Geometry check sheet. Reference: the model listing, model coordinates, mm. Face numbers are marked on the shaded views. A direction names the side the tool comes from. Round coordinates to 2 decimals unless told otherwise and drop trailing zeros. Loops run counter-clockwise (first coordinate to the right, second up) from the corner with the lowest first, then second, coordinate; pieces in that order, holes last. Notation, with made-up numbers: M -17,36 L 2,36 A21 cw 2,53 Z; hole C 40.25,1.5 d3. An arc over 180 degrees is marked long. Write item = value, one per line.
from build123d import *

# Parameters (mm, degrees)
BOSS_EXTRUDE5_DEPTH    = 10
BOSS_EXTRUDE5_2_DEPTH  = 10
BOSS_EXTRUDE5_3_DEPTH  = 10
BOSS_EXTRUDE5_4_DEPTH  = 10
BOSS_EXTRUDE5_5_DEPTH  = 10
BOSS_EXTRUDE5_6_DEPTH  = 10
BOSS_EXTRUDE5_7_DEPTH  = 10
BOSS_EXTRUDE5_8_DEPTH  = 10
BOSS_EXTRUDE5_9_DEPTH  = 10
BOSS_EXTRUDE5_10_DEPTH = 10
BOSS_EXTRUDE5_11_DEPTH = 10
BOSS_EXTRUDE5_12_DEPTH = 10
SKETCH5_W              = 13.85640646
SKETCH5_H              = 26
SKETCH5_W_2            = 26.92820323
SKETCH5_H_2            = 12
BOSS_EXTRUDE8_DEPTH    = 76.2
BOSS_EXTRUDE9_REACH    = 266.711
SKETCH9_W              = 6.35
SKETCH9_H              = 128.000000074
SKETCH9_W_2            = 11.02820323
BOSS_EXTRUDE10_DEPTH   = 152.4
SKETCH11_W             = 226.92820323
SKETCH11_H             = 76.2
BOSS_EXTRUDE11_DEPTH   = 6.35


with BuildPart() as part:
    # Sketch2 → Boss-Extrude5 (new body)
    with BuildSketch(Plane.XY):
        Polygon((-111.732050808, 13), (-113.464101615, 10), (-111.732050808, 7), (-108.267949192, 7), (-106.535898385, 10), (-108.267949192, 13), align=None)
    extrude(amount=-BOSS_EXTRUDE5_DEPTH)



with BuildPart() as body_2:
    # Sketch2 → Boss-Extrude5 2 (new body)
    with BuildSketch(Plane.XY):
        Polygon((-111.732050808, 23), (-113.464101615, 20), (-111.732050808, 17), (-108.267949192, 17), (-106.535898385, 20), (-108.267949192, 23), align=None)
    extrude(amount=-BOSS_EXTRUDE5_2_DEPTH)


with BuildPart() as body_3:
    # Sketch2 → Boss-Extrude5 3 (new body)
    with BuildSketch(Plane.XY):
        Polygon((-111.732050808, 33), (-113.464101615, 30), (-111.732050808, 27), (-108.267949192, 27), (-106.535898385, 30), (-108.267949192, 33), align=None)
    extrude(amount=-BOSS_EXTRUDE5_3_DEPTH)


with BuildPart() as body_4:
    # Sketch2 → Boss-Extrude5 4 (new body)
    with BuildSketch(Plane.XY):
        Polygon((111.732050808, 27), (113.464101615, 30), (111.732050808, 33), (108.267949192, 33), (106.535898385, 30), (108.267949192, 27), align=None)
    extrude(amount=-BOSS_EXTRUDE5_4_DEPTH)


with BuildPart() as body_5:
    # Sketch2 → Boss-Extrude5 5 (new body)
    with BuildSketch(Plane.XY):
        Polygon((111.732050808, 17), (113.464101615, 20), (111.732050808, 23), (108.267949192, 23), (106.535898385, 20), (108.267949192, 17), align=None)
    extrude(amount=-BOSS_EXTRUDE5_5_DEPTH)


with BuildPart() as body_6:
    # Sketch2 → Boss-Extrude5 6 (new body)
    with BuildSketch(Plane.XY):
        Polygon((111.732050808, 7), (113.464101615, 10), (111.732050808, 13), (108.267949192, 13), (106.535898385, 10), (108.267949192, 7), align=None)
    extrude(amount=-BOSS_EXTRUDE5_6_DEPTH)


with BuildPart() as body_7:
    # Sketch2 → Boss-Extrude5 7 (new body)
    with BuildSketch(Plane.XY):
        Polygon((61.732050808, 107), (63.464101615, 110), (61.732050808, 113), (58.267949192, 113), (56.535898385, 110), (58.267949192, 107), align=None)
    extrude(amount=-BOSS_EXTRUDE5_7_DEPTH)


with BuildPart() as body_8:
    # Sketch2 → Boss-Extrude5 8 (new body)
    with BuildSketch(Plane.XY):
        Polygon((51.732050808, 107), (53.464101615, 110), (51.732050808, 113), (48.267949192, 113), (46.535898385, 110), (48.267949192, 107), align=None)
    extrude(amount=-BOSS_EXTRUDE5_8_DEPTH)


with BuildPart() as body_9:
    # Sketch2 → Boss-Extrude5 9 (new body)
    with BuildSketch(Plane.XY):
        Polygon((41.732050808, 107), (43.464101615, 110), (41.732050808, 113), (38.267949192, 113), (36.535898385, 110), (38.267949192, 107), align=None)
    extrude(amount=-BOSS_EXTRUDE5_9_DEPTH)


with BuildPart() as body_10:
    # Sketch2 → Boss-Extrude5 10 (new body)
    with BuildSketch(Plane.XY):
        Polygon((-38.267949192, 107), (-36.535898385, 110), (-38.267949192, 113), (-41.732050808, 113), (-43.464101615, 110), (-41.732050808, 107), align=None)
    extrude(amount=-BOSS_EXTRUDE5_10_DEPTH)


with BuildPart() as body_11:
    # Sketch2 → Boss-Extrude5 11 (new body)
    with BuildSketch(Plane.XY):
        Polygon((-48.267949192, 107), (-46.535898385, 110), (-48.267949192, 113), (-51.732050808, 113), (-53.464101615, 110), (-51.732050808, 107), align=None)
    extrude(amount=-BOSS_EXTRUDE5_11_DEPTH)


with BuildPart() as body_12:
    # Sketch2 → Boss-Extrude5 12 (new body)
    with BuildSketch(Plane.XY):
        Polygon((-58.267949192, 107), (-56.535898385, 110), (-58.267949192, 113), (-61.732050808, 113), (-63.464101615, 110), (-61.732050808, 107), align=None)
    extrude(amount=-BOSS_EXTRUDE5_12_DEPTH)


with BuildPart() as part_1:
    add(part.part)

    add(body_2.part)  # Boss-Extrude8 merges body 2

    add(body_3.part)  # Boss-Extrude8 merges body 3

    add(body_4.part)  # Boss-Extrude8 merges body 4

    add(body_5.part)  # Boss-Extrude8 merges body 5

    add(body_6.part)  # Boss-Extrude8 merges body 6

    add(body_7.part)  # Boss-Extrude8 merges body 7

    add(body_8.part)  # Boss-Extrude8 merges body 8

    add(body_9.part)  # Boss-Extrude8 merges body 9

    add(body_10.part)  # Boss-Extrude8 merges body 10

    add(body_11.part)  # Boss-Extrude8 merges body 11

    add(body_12.part)  # Boss-Extrude8 merges body 12
    # Sketch5 → Boss-Extrude8 (add)
    with BuildSketch(Plane.XY):
        with Locations((-106.535898385, 20)):
            Rectangle(SKETCH5_W, SKETCH5_H)
        with Locations((-50, 107)):
            Rectangle(SKETCH5_W_2, SKETCH5_H_2)
        with Locations((50, 107)):
            Rectangle(SKETCH5_W_2, SKETCH5_H_2)
        with Locations((106.535898385, 20)):
            Rectangle(SKETCH5_W, SKETCH5_H)
    extrude(amount=BOSS_EXTRUDE8_DEPTH)

    # Boss-Extrude9: up to this face of the body (flat: up to its plane)
    boss_extrude9_end = Plane(part_1.part.faces().sort_by_distance((-113.464101615, 20, 38.1))[0])
    # Sketch8 → Boss-Extrude9 (add, up to the picked face)
    with BuildSketch(Plane(origin=(113.464101615, 0, 0), x_dir=(0, 0, -1), z_dir=(1, 0, 0)), mode=Mode.PRIVATE) as boss_extrude9_sk1:
        Polygon((-76.2, 113), (-76.2, -15.000000074), (-114.3, -15.000000074), align=None)
    boss_extrude9_tool1 = split(extrude(boss_extrude9_sk1.sketch, amount=-BOSS_EXTRUDE9_REACH, mode=Mode.PRIVATE), bisect_by=boss_extrude9_end, keep=Keep.BOTH, mode=Mode.PRIVATE)
    add(boss_extrude9_tool1.solids().sort_by(Axis((113.464102, 27.666667, 88.9), (-1, 0, 0)))[0])

    # Sketch9 → Boss-Extrude10 (add)
    with BuildSketch(Plane(origin=(0, 0, 76.2), x_dir=(-1, 0, 0), z_dir=(0, 0, -1))):
        with Locations((-110.289101615, 48.999999963)):
            Rectangle(SKETCH9_W, SKETCH9_H)
        with Locations((110.289101615, 48.999999963)):
            Rectangle(SKETCH9_W, SKETCH9_H)
        with Locations((0, 48.999999963)):
            Rectangle(SKETCH9_W_2, SKETCH9_H)
    extrude(amount=-BOSS_EXTRUDE10_DEPTH)

    # Sketch11 → Boss-Extrude11 (add)
    with BuildSketch(Plane(origin=(0, 113, 0), x_dir=(1, 0, 0), z_dir=(0, 1, 0))):
        with Locations((0, -190.5)):
            Rectangle(SKETCH11_W, SKETCH11_H)
    extrude(amount=-BOSS_EXTRUDE11_DEPTH)


solid = part_1.part
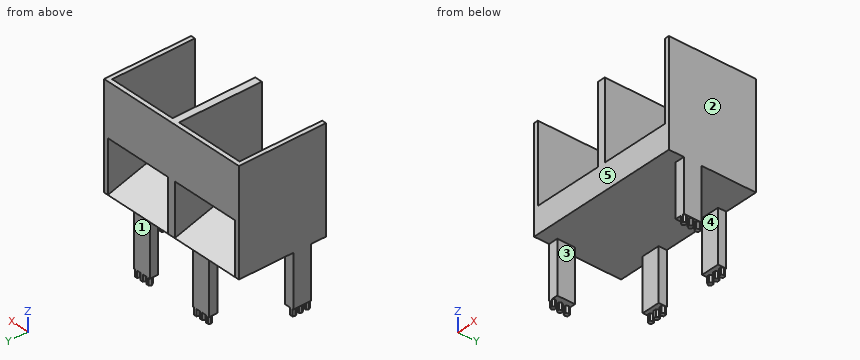
(1) Sectioned sample at D-D on y = 82.5. Record the cut outline in (x, z).
Result set:
outline = M -113.46,76.2 L 113.46,76.2 L 113.46,228.6 L 107.11,228.6 L 107.11,85.28 L 5.51,85.28 L 5.51,228.6 L -5.51,228.6 L -5.51,85.28 L -107.11,85.28 L -107.11,228.6 L -113.46,228.6 Z
(2) Sectioned sample at A-A on x = 17.5. Record the cut outline in (y, z), then the cut area to 3 significant figures.
Result set:
outline = M -15,76.2 L 113,76.2 L -15,114.3 Z; M 106.65,152.4 L 113,152.4 L 113,228.6 L 106.65,228.6 Z
area = 2,920 mm2
(3) Depth check by flat-ended pin: pin 1 Ø3 at (x, y) = (44.5, 111) entering from -Z; pin 2 Ø23 at (x, z) = (-61, 193.5) entering from -Y; pin 3 Ø8 at (x, z) = (-55.5, 54) entering from -Y; pin 4 Ø3 at (x, y) = (-50, 79.5) entering from +Z. Enter the tip coordinate at first touch or a pass-through.
Result set:
pin_1 = -10
pin_2 = 106.65
pin_3 = 101
pin_4 = 86.62
(4) Sectioned sample at C-C on z = 33. Record the cut outline in (x, y).
Result set:
outline = M -113.46,7 L -99.61,7 L -99.61,33 L -113.46,33 Z; M -63.46,101 L -36.54,101 L -36.54,113 L -63.46,113 Z; M 36.54,101 L 63.46,101 L 63.46,113 L 36.54,113 Z; M 99.61,7 L 113.46,7 L 113.46,33 L 99.61,33 Z
(5) Sectioned sample at B-B on z = 142.5. Record the cut outline in (x, y).
Result set:
outline = M -113.46,-15 L -107.11,-15 L -107.11,113 L -113.46,113 Z; M -5.51,-15 L 5.51,-15 L 5.51,113 L -5.51,113 Z; M 107.11,-15 L 113.46,-15 L 113.46,113 L 107.11,113 Z
(6) Release check for a two-part mould opening along X. For the marked faces 1, 2 and 3 record: released by +X, released by -X, zero draft, split by the parting line, or undercut.
Result set:
face_1 = zero draft
face_2 = released by +X
face_3 = undercut
(7) Tool access check on the marked faces 4 and 5. Record the directions out of +Z, -Z, +X, -X, +Y, -Y that give a thin tool (end or side, any length) a straight path to the whole face; none if there is none.
Result set:
face_4 = -Z, +X, -X, -Y
face_5 = +Z, -Z, +X, -X, -Y
(8) Material ranges on line 1 along X through (y, z) = (60, 192.5); line 2 along Y through (x, z) = (-25, 192); line 3 along Y through (x, z) = (-38, 37), recorded low to high. Write a range as from..to.
Result set:
line_1 = -113.46..-107.11, -5.51..5.51, 107.11..113.46
line_2 = 106.65..113
line_3 = 101..113
